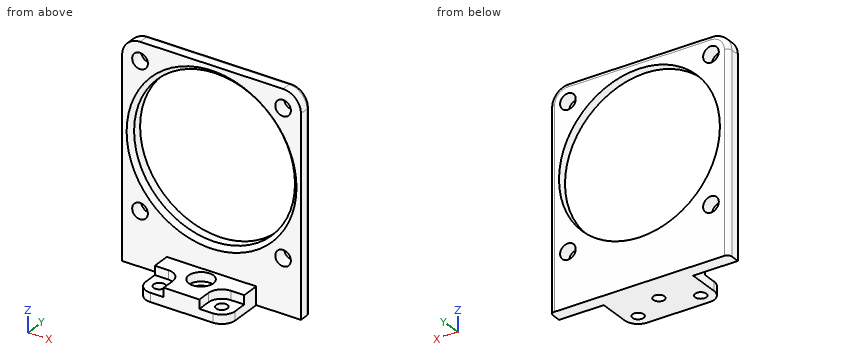
```python
from build123d import *

# Parameters (mm, degrees)
F0_W     = 40
F0_H     = 48
F0_R     = 1.75
F0_R_2   = 18
F1_DEPTH = 3
F2_W     = 20
F2_H     = 4
F3_DEPTH = 13
F4_R     = 1.25
F5_DEPTH = 25
F6_W     = 6
F6_H     = 6
F6_R     = 2.75
F7_DEPTH = 2
F8_R     = 4
F9_R     = 3
F10_SIZE = 1
F11_R    = 1


with BuildPart() as f1:
    # F0 (on Front) → F1 (new body)
    with BuildSketch(Plane.XZ):
        with Locations((0, 24)):
            Rectangle(F0_W, F0_H)
        with Locations((-16, 11.902926147)):
            Circle(F0_R, mode=Mode.SUBTRACT)
        with Locations((16, 11.902926147)):
            Circle(F0_R, mode=Mode.SUBTRACT)
        with Locations((-16, 43.902926147)):
            Circle(F0_R, mode=Mode.SUBTRACT)
        with Locations((0, 27.902926147)):
            Circle(F0_R_2, mode=Mode.SUBTRACT)
        with Locations((16, 43.902926147)):
            Circle(F0_R, mode=Mode.SUBTRACT)
    extrude(amount=F1_DEPTH)

    # F2 (on Front) → F3 (join)
    with BuildSketch(Plane.XZ):
        with Locations((0, 2)):
            Rectangle(F2_W, F2_H)
    extrude(amount=F3_DEPTH)

    # F4 (on Top) → F5 (cut)
    with BuildSketch(Plane.XY):
        with Locations((0, -6.5)):
            Circle(F4_R)
        with Locations((-7, -10)):
            Circle(F4_R)
        with Locations((7, -10)):
            Circle(F4_R)
    extrude(amount=F5_DEPTH, mode=Mode.SUBTRACT)

    # F6 (on face) → F7 (cut)
    with BuildSketch(Plane.XY.offset(4)):
        with Locations((-7, -10)):
            Rectangle(F6_W, F6_H)
        with Locations((7, -10)):
            Rectangle(F6_W, F6_H)
        with Locations((0, -6.5)):
            Circle(F6_R)
    extrude(amount=-F7_DEPTH, mode=Mode.SUBTRACT)

    # F8
    f8_edges = [f1.edges().sort_by_distance(p)[0] for p in [
        (20, -1.5, 48),
        (-20, -1.5, 48),
    ]]
    fillet(f8_edges, radius=F8_R)

    # F9
    f9_edges = [f1.edges().sort_by_distance(p)[0] for p in [
        (4, -7, 3),
        (10, -13, 1),
        (-4, -7, 3),
        (-10, -13, 1),
    ]]
    fillet(f9_edges, radius=F9_R)

    # F10
    f10_edges = [f1.edges().sort_by_distance(p)[0] for p in [
        (-18, -3, 27.902926),
    ]]
    chamfer(f10_edges, length=F10_SIZE)

    # F11
    f11_edges = [f1.edges().sort_by_distance(p)[0] for p in [
        (20, 0, 22),
    ]]
    fillet(f11_edges, radius=F11_R)


solid = f1.part
```
Input: part model. Units: mm. Frame: model coordinates. Give positions to 0.01 mm unless a question says otherwise; leave off trailing zeros. Order: outer loops, then holes, each group sorted by start corner. A loop starts at its lowest first (then second) coordinate and runs counter-clockwise, first axis right, second up.
1. Section B-B on z = 8. Return the cut outline in (x, y).
Derived:
outline: (-20, -3) - (20, -3) - (20, -1) arc R1 ccw to (19, 0) - (-19, 0) arc R1 ccw to (-20, -1) - close
2. Material intervals for L1, parallel to X at y = -10, z = 0.8; L2, parallel to Z at x = 0, y = -0.95; L3, parallel to Y at x = -7, z = 1, sorted ascending.
Derived:
L1: x = -10 to -8.25, -5.75 to 5.75, 8.25 to 10
L2: z = 0 to 9.9, 45.9 to 48
L3: y = -13 to -11.25, -8.75 to 0
3. Section A-A on x = 0. Return the cut outline in (y, z), and give its area (3 significant figures).
Derived:
outline: (-13, 0) - (-7.75, 0) - (-7.75, 2) - (-9.25, 2) - (-9.25, 4) - (-13, 4) - close; (-5.25, 0) - (0, 0) - (0, 9.9) - (-2, 9.9) - (-3, 8.9) - (-3, 4) - (-3.75, 4) - (-3.75, 2) - (-5.25, 2) - close; (-3, 46.9) - (-2, 45.9) - (0, 45.9) - (0, 47) arc R1 ccw to (-1, 48) - (-3, 48) - close
area: 58.8 mm2
4. Pin query (flat end, axial travel): pin 1 (20 mm diameter, centred on x = -3.5, z = 28, fed in from -Y); pin 2 (0.6 mm diameter, centred on y = -11.5, z = 3, fed in from +X); pin 3 (1.2 mm diameter, centred on y = -5, z = 3, fed in from -X); pin 4 (2 mm diameter, centred on x = -8.5, z = 2.5, fed in from -Y). Return the tip coordinate at first contact, or that it passes through.
Derived:
pin 1: passes through
pin 2: stops at x = 4
pin 3: stops at x = -10
pin 4: stops at y = -12.93
